```python
from build123d import *

# Parameters (mm, degrees)
SKETCH3_R          = 1
CUT_EXTRUDE1_DEPTH = 4
SKETCH4_R          = 2.25
CUT_EXTRUDE2_DEPTH = 1


with BuildPart() as part:
    # Sketch1 → Revolve1 (revolve)
    with BuildSketch(Plane.XY):
        Polygon((0, 0), (8, 0), (8, 3), (2, 3), (2, 14), (0, 14), align=None)
    revolve(axis=Axis((0, 14, 0), (0, -1, 0)))

    # Sketch3 → Cut-Extrude1 (cut, through all)
    with BuildSketch(Plane(origin=(0, 3, 0), x_dir=(1, 0, 0), z_dir=(0, 1, 0))):
        with Locations((0, 4.5)):
            Circle(SKETCH3_R)
        with Locations((4.5, 0)):
            Circle(SKETCH3_R)
        with Locations((0, -4.5)):
            Circle(SKETCH3_R)
        with Locations((-4.5, 0)):
            Circle(SKETCH3_R)
    extrude(amount=-CUT_EXTRUDE1_DEPTH, mode=Mode.SUBTRACT)

    # Sketch4 → Cut-Extrude2 (cut)
    with BuildSketch(Plane(origin=(0, 3, 0), x_dir=(1, 0, 0), z_dir=(0, 1, 0))):
        with Locations((0, 4.5)):
            Circle(SKETCH4_R)
        with Locations((4.5, 0)):
            Circle(SKETCH4_R)
        with Locations((0, -4.5)):
            Circle(SKETCH4_R)
        with Locations((-4.5, 0)):
            Circle(SKETCH4_R)
    extrude(amount=-CUT_EXTRUDE2_DEPTH, mode=Mode.SUBTRACT)


solid = part.part
```
Work out the finished part from the listing and answer in its coordinate system (mm). A direction names the side the tool comes from. Round coordinates to 2 decimals unless told otherwise and drop trailing zeros. Write each loop counter-clockwise with the first axis right and the second up, starting at its lowest first coordinate (ties: lowest second). Pieces come first, ordered by that corner, then holes. Notation, with made-up numbers: (-39.5, 17) -> (2.5, 17) arc R26 cw to (2.5, 39) -> close; hole circle Ø11 at (-23, 65). An arc over 180 degrees is marked (long way). Write each question's results on one line, items separated by ' | '.
1) The part is cut by section D-D (z = 4.5). Write down the section's boundary in (x, y), and give its area (3 significant figures).
Findings:
outline: (-6.61, 0) -> (-1, 0) -> (-1, 2) -> (-2.25, 2) -> (-2.25, 3) -> (-6.61, 3) -> close; (1, 0) -> (6.61, 0) -> (6.61, 3) -> (2.25, 3) -> (2.25, 2) -> (1, 2) -> close | area: 31.2 mm²
2) Consider line 1 along Y through (x, z) = (-1.75, 3.5); line 2 along Z through (x, y) = (4.5, 2.4); line 3 along X through (y, z) = (1.3, 4.5). Determine where each line is inside the solid, lowest interval first. Write a range as [from, to].
Findings:
line 1: y = [0, 2] | line 2: z = [-6.61, -2.25], [2.25, 6.61] | line 3: x = [-6.61, -1], [1, 6.61]
3) Flat-ended cylindrical pins translate along their axes: pin 1 (2 mm diameter, centred on y = 9.5, z = 1.5, fed in from +X); pin 2 (2.5 mm diameter, centred on x = 0, z = -4.5, fed in from +Y); pin 3 (5 mm diameter, centred on x = 0.5, y = 7, fed in from -Z); pin 4 (4 mm diameter, centred on x = 0, z = -4.5, fed in from -Y). Find the tip coordinate at first contact, or state that the pin passes through.
Findings:
pin 1: stops at x = 1.94 | pin 2: stops at y = 2 | pin 3: stops at z = -2 | pin 4: stops at y = 0
4) The part is cut by section B-B (x = -5). Write down the section's boundary in (y, z) (3 decimals), and give its area (3 significant figures).
Findings:
outline: (0, -6.245) -> (3, -6.245) -> (3, -2.194) -> (2, -2.194) -> (2, -0.866) -> (0, -0.866) -> close; (0, 0.866) -> (2, 0.866) -> (2, 2.194) -> (3, 2.194) -> (3, 6.245) -> (0, 6.245) -> close | area: 29.6 mm²
5) Which of the six approach directions +Z, -Z, +X, -X, +Y, -Y give full straight-line access (tool end or side, diameter ignored) to faces 1 (the cylindrical face through (-5.3, 1, 0.6)), 2 (the flat face through (-6, 2, 0))?
Findings:
face 1: +Y, -Y | face 2: +Y
6) For a pull along Z with two mould halves and no side action, classify faces 3 (the cylindrical face through (6.646, 2.507, -0.676)), 4 (the flat face through (0, 0, 0)), 5 (the cylindrical face through (-0.13, 1.01, -5.49)), 6 (the cylindrical face through (-1.73, 1.52, -7.81)) as +Z half, -Z half, draft (parallel to the pull), parting line (faces both ways), or undercut.
Findings:
face 3: undercut | face 4: draft | face 5: undercut | face 6: parting line
7) The part is cut by section C-C (y = 1.5). Write down the section's boundary in (x, z), and give its area (3 significant figures).
Findings:
outline: circle Ø16 at (0, 0); hole circle Ø2 at (-4.5, 0); hole circle Ø2 at (0, -4.5); hole circle Ø2 at (0, 4.5); hole circle Ø2 at (4.5, 0) | area: 188 mm²
8) The part is cut by section A-A (z = 0). Write down the section's boundary in (x, y), and give its area (3 significant figures).
Findings:
outline: (-8, 0) -> (-5.5, 0) -> (-5.5, 2) -> (-6.75, 2) -> (-6.75, 3) -> (-8, 3) -> close; (-3.5, 0) -> (3.5, 0) -> (3.5, 2) -> (2.25, 2) -> (2.25, 3) -> (2, 3) -> (2, 14) -> (-2, 14) -> (-2, 3) -> (-2.25, 3) -> (-2.25, 2) -> (-3.5, 2) -> close; (5.5, 0) -> (8, 0) -> (8, 3) -> (6.75, 3) -> (6.75, 2) -> (5.5, 2) -> close | area: 75.0 mm²
